Can you work these out from the model? Positions are in its coordinate system, mm. A direction names the side the tool comes from. Coordinates: 2 decimals unless noted, no trailing zeros. Loops run counter-clockwise (first coordinate to the right, second up) from the corner with the lowest first, then second, coordinate; pieces in that order, holes last. Notation, with made-up numbers: (-31, 7) -> (1, 7) arc R9 ccw to (1, 16) -> close; hole circle Ø1 at (-26, 77.25). An arc over 180 degrees is marked (long way). Put each result on its own line as item: value. Start each with the question number.
Item 1: If we section it at A-A on y = -35.5: Please give me the cut outline in (x, z), plus the area to 3 significant figures.
Item 2: We'd pull the mould along Y, two halves only. Please class faces 6 (the flat face through (-32, -37.5, 2)), 7 (the flat face through (0, -90.5, 1)), 8 (the cylindrical face through (-23.434, 38.452, 1.479)), 9 (the flat face through (-33, -50, 2)): pulls with the +Y half, pulls with the -Y half, needs draft (parallel to the pull), parting line crosses it, or undercut.
Item 3: Will these pins go through, and if not, where does the flat tip stop? P1, Ø1.5, axis at y = -40, z = 1.5, coming from the -X side; P2, Ø1.5, axis at y = -92, z = 1.5, coming from the +X side; P3, Ø0.9, axis at x = -31.5, z = 1.5, coming from the +Y side; P4, Ø3.5, axis at x = 0, y = -35.5, coming from the +Z side.
Item 4: For faces 1 (the flat face through (-33, -10, 2)), 2 (the flat face through (-30, 40, 1)), 3 (the flat face through (-22.5, 92, 2)), 4 (the flat face through (22.5, 92, 2)), 5 (the flat face through (-7.5, -92, 2)), which set-ups out of +Z, -Z, +X, -X, +Y, -Y let a thin tool reach every point of the face, with its end or its side?
Item 5: Please list where these lines run through material, in increasing order: L1, parallel to X at y = -83, z = 1.1; L2, parallel to X at y = -81, z = 2.75. Write a range as from..to.
Item 6: If we section it at B-B on z = 2.2: State how many separate pieces and enclosed holes the cut face has, plus the area to 3 significant figures.
Autodesk Inventor part; units mm, degrees
ref_plane "YZ Plane" through (0, 0, 0) normal (1, 0, 0) x (0, 1, 0)
ref_plane "XZ Plane" through (0, 0, 0) normal (0, 1, 0) x (-1, 0, 0)
ref_plane "XY Plane" through (0, 0, 0) normal (0, 0, 1) x (1, 0, 0)
sketch "Sketch1" plane through (0, 0, 0) normal (0, 0, 1) x (1, 0, 0)
  line L0 (-30, -90.5) -> (30, -90.5)
  line L1 (30, -90.5) -> (30, 90.5)
  line L2 (30, 90.5) -> (-30, 90.5)
  line L3 (-30, 90.5) -> (-30, -90.5)
  line L4 (-30, -90.5) -> (30, 90.5) construction
  line L5 (30, -90.5) -> (-30, 90.5) construction
  circle A0 centre (-23, 60.5) radius 2
  circle A1 centre (-23, 36.5) radius 2
  circle A2 centre (-23, 12.5) radius 2
  circle A3 centre (-23, -11.5) radius 2
  circle A4 centre (-23, -35.5) radius 2
  circle A5 centre (-23, -59.5) radius 2
  circle A6 centre (-23, -83.5) radius 2
  circle A7 centre (0, 60.5) radius 2
  circle A8 centre (0, 36.5) radius 2
  circle A9 centre (0, 12.5) radius 2
  circle A10 centre (0, -11.5) radius 2
  circle A11 centre (0, -35.5) radius 2
  circle A12 centre (0, -59.5) radius 2
  circle A13 centre (0, -83.5) radius 2
  circle A14 centre (23, 60.5) radius 2
  circle A15 centre (23, 36.5) radius 2
  circle A16 centre (23, 12.5) radius 2
  circle A17 centre (23, -11.5) radius 2
  circle A18 centre (23, -35.5) radius 2
  circle A19 centre (23, -59.5) radius 2
  circle A20 centre (23, -83.5) radius 2
  point P0 (0, 0)
  dimension "d0" = 60
  dimension "d1" = 181
  dimension "d2" = 4
  dimension "d3" = 30
  dimension "d6" = 24
  dimension "d9" = 23
  dimension "d12" = 7
extrude "Extrusion1" add sketch "Sketch1" along normal blind 3
sketch "Sketch2" plane through (0, 0, 3) normal (0, 0, 1) x (1, 0, 0)
  line L0 (-30, 90.5) -> (-30, -90.5)
  line L1 (-30, 77.5) -> (-33, 77.5)
  line L2 (-33, 77.5) -> (-33, 62.5)
  line L3 (-33, 62.5) -> (-30, 62.5)
  line L4 (-30, 62.5) -> (-30, 77.5)
  line L5 (-30, 57.5) -> (-33, 57.5)
  line L6 (-33, 57.5) -> (-33, 42.5)
  line L7 (-33, 42.5) -> (-30, 42.5)
  line L8 (-30, 42.5) -> (-30, 57.5)
  line L9 (-30, 37.5) -> (-33, 37.5)
  line L10 (-33, 37.5) -> (-33, 22.5)
  line L11 (-33, 22.5) -> (-30, 22.5)
  line L12 (-30, 22.5) -> (-30, 37.5)
  line L13 (-30, 17.5) -> (-33, 17.5)
  line L14 (-33, 17.5) -> (-33, 2.5)
  line L15 (-33, 2.5) -> (-30, 2.5)
  line L16 (-30, 2.5) -> (-30, 17.5)
  line L17 (-30, -2.5) -> (-33, -2.5)
  line L18 (-33, -2.5) -> (-33, -17.5)
  line L19 (-33, -17.5) -> (-30, -17.5)
  line L20 (-30, -17.5) -> (-30, -2.5)
  line L21 (-30, -22.5) -> (-33, -22.5)
  line L22 (-33, -22.5) -> (-33, -37.5)
  line L23 (-33, -37.5) -> (-30, -37.5)
  line L24 (-30, -37.5) -> (-30, -22.5)
  line L25 (-30, -42.5) -> (-33, -42.5)
  line L26 (-33, -42.5) -> (-33, -57.5)
  line L27 (-33, -57.5) -> (-30, -57.5)
  line L28 (-30, -57.5) -> (-30, -42.5)
  line L29 (-30, -62.5) -> (-33, -62.5)
  line L30 (-33, -62.5) -> (-33, -77.5)
  line L31 (-33, -77.5) -> (-30, -77.5)
  line L32 (-30, -77.5) -> (-30, -62.5)
  point P0 (0, 0)
  dimension "d15" = 3
  dimension "d16" = 15
  dimension "d17" = 13
  dimension "d20" = 20
extrude "Extrusion2" add sketch "Sketch2" against normal blind 3
sketch "Sketch3" plane through (0, 0, 3) normal (0, 0, 1) x (1, 0, 0)
  line L0 (30, 90.5) -> (-30, 90.5)
  line L1 (-22.5, 90.5) -> (-7.5, 90.5)
  line L2 (-7.5, 90.5) -> (-7.5, 93.5)
  line L3 (-7.5, 93.5) -> (-22.5, 93.5)
  line L4 (-22.5, 93.5) -> (-22.5, 90.5)
  line L5 (-22.5, -93.5) -> (-7.5, -93.5)
  line L6 (-7.5, -93.5) -> (-7.5, -90.5)
  line L7 (-7.5, -90.5) -> (-22.5, -90.5)
  line L8 (-22.5, -90.5) -> (-22.5, -93.5)
  line L9 (7.5, 90.5) -> (22.5, 90.5)
  line L10 (22.5, 90.5) -> (22.5, 93.5)
  line L11 (22.5, 93.5) -> (7.5, 93.5)
  line L12 (7.5, 93.5) -> (7.5, 90.5)
  line L13 (7.5, -93.5) -> (22.5, -93.5)
  line L14 (22.5, -93.5) -> (22.5, -90.5)
  line L15 (22.5, -90.5) -> (7.5, -90.5)
  line L16 (7.5, -90.5) -> (7.5, -93.5)
  line L17 (-30, 90.5) -> (-30, 77.5)
  point P0 (0, 0)
  dimension "d27" = 15
  dimension "d28" = 3
  dimension "d31" = 184
  dimension "d34" = 30
  dimension "d37" = 7.5
extrude "Extrusion3" add sketch "Sketch3" against normal blind 3
equation "\"BendRadius\" = Thickness"
equation "\"BendReliefWidth\" = Thickness"
equation "\"BendReliefDepth\" = 0.5 * Thickness"
equation "\"CornerReliefSize\" = 4 * Thickness"
equation "\"MinimumRemnant\" = 2 * Thickness"
equation "\"TransitionRadius\" = BendRadius"
equation "\"JacobiRadiusSize\" = BendRadius"
equation "\"GapSize\" = Thickness"
properties part number "2 binnen zijplaat"
Solutions:
1. outline: (-33, 0) -> (-25, 0) -> (-25, 3) -> (-33, 3) -> close; (-21, 0) -> (-2, 0) -> (-2, 3) -> (-21, 3) -> close; (2, 0) -> (21, 0) -> (21, 3) -> (2, 3) -> close; (25, 0) -> (30, 0) -> (30, 3) -> (25, 3) -> close
1. area: 153 mm^2
2. face 6: undercut
2. face 7: pulls with the -Y half
2. face 8: undercut
2. face 9: needs draft
3. P1: x = -30
3. P2: x = 22.5
3. P3: y = 77.5
3. P4: through
4. face 1: +Z, -Z, -X, +Y, -Y
4. face 2: +Z, -Z, -X
4. face 3: +Z, -Z, -X, +Y
4. face 4: +Z, -Z, +X, +Y
4. face 5: +Z, -Z, -Y
5. L1: -30..-24.94, -21.06..-1.94, 1.94..21.06, 24.94..30
5. L2: -30..30
6. separate pieces: 1
6. enclosed holes: 21
6. area: 11,100 mm^2
